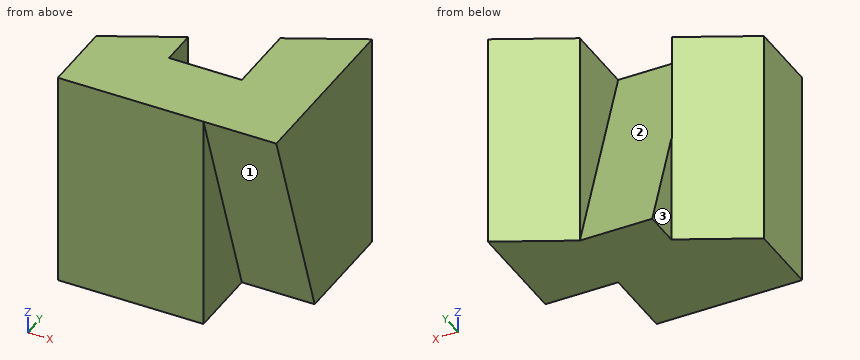
from build123d import *

# Parameters (mm, degrees)
SKETCH1_W           = 6
SKETCH1_H           = 6
BOSS_EXTRUDE1_DEPTH = 5
CUT_EXTRUDE12_DEPTH = 12
CUT_EXTRUDE13_DEPTH = 1
CUT_EXTRUDE14_DEPTH = 2


with BuildPart() as part:
    # Sketch1 → Boss-Extrude1 (new body)
    with BuildSketch(Plane(origin=(0, 0, 0), x_dir=(1, 0, 0), z_dir=(0, 1, 0))):
        Rectangle(SKETCH1_W, SKETCH1_H)
    extrude(amount=BOSS_EXTRUDE1_DEPTH)

    # Sketch11 → Cut-Extrude12 (cut)
    with BuildSketch(Plane.XY.offset(3)):
        Polygon((-3, 5), (-3, 2), (-0.98808733, 3.005956335), (-0.98808733, 4), (0.98808733, 4), (0.98808733, 3.994043665), (3, 5), align=None)
    extrude(amount=-CUT_EXTRUDE12_DEPTH, mode=Mode.SUBTRACT)

    # Sketch12 → Cut-Extrude13 (cut, symmetric)
    with BuildSketch(Plane(origin=(0, 0, 0), x_dir=(0, 0, -1), z_dir=(1, 0, 0))):
        Polygon((3, 4), (-3, 2), (-3, 3.005956335), (-3, 4), align=None)
    extrude(amount=CUT_EXTRUDE13_DEPTH, both=True, mode=Mode.SUBTRACT)

    # Sketch13 → Cut-Extrude14 (cut)
    with BuildSketch(Plane(origin=(3, 0, 0), x_dir=(0, 0, -1), z_dir=(1, 0, 0))):
        Polygon((3, 2), (-3, 0), (3, 0), align=None)
    extrude(amount=-CUT_EXTRUDE14_DEPTH, mode=Mode.SUBTRACT)


solid = part.part
Source: CAD feature listing. Evaluate the final solid. Frame: model axes, mm. Face numbers are marked on the shaded views. A direction names the side the tool comes from. Round coordinates to 2 decimals unless told otherwise and drop trailing zeros. Write each loop counter-clockwise with the first axis right and the second up, starting at its lowest first coordinate (ties: lowest second). Pieces come first, ordered by that corner, then holes. Notation, with made-up numbers: (24, 82) - (57, 82) arc R11 ccw to (57, 96) - close; hole circle Ø9 at (69, 53). An arc over 180 degrees is marked (long way). Use CSV: the item, a comma, the result in double quotes. Start each with the question number.
(1) Cut plane C-C, the plane x = 1.5. Return loops of the section in (y, z).
(2) First-contact query: pin 1 Ø1.1 at (y, z) = (3.5, -2) entering from -X; pin 2 Ø1.5 at (x, z) = (1.5, -1.5) entering from +Y (3 decimals); pin 3 Ø2 at (x, z) = (1.5, -1.5) entering from +Y. Flat tips, straight axial feed; report the tip coordinate or a pass-through.
(3) Set-up query: the marked faces 1, 2 and 3. Return all of +Z, -Z, +X, -X, +Y, -Y with unobstructed straight access to the full face (end or side cutting, diameter ignored); none if empty.
(4) Cut plane A-A, the plane y = 2.8. Return loops of the section in (x, z).
(5) Cut plane B-B, the plane z = 1.25. Return loops of the section in (x, y), and give its area (3 significant figures).
(6) Material intervals for probe 1 along X at (y, z) = (1.2, -2); probe 2 along X at (y, z) = (3.4, -2.25); probe 3 along X at (y, z) = (2.8, 2.5), sorted ascending. Write a range as [from, to].
(7) Cut plane D-D, the plane y = 0.55. Return loops of the section in (x, z), and give its area (3 significant figures).
Geometry says:
1,outline,"(0, 3) - (2, -3) - (4.25, -3) - (4.25, 3) - close"
2,pin 1,"x = -1.1"
2,pin 2,"y = 4.625"
2,pin 3,"y = 4.75"
3,face 1,"-Z, +X, -Y"
3,face 2,"+Z, +Y"
3,face 3,"+Z, -Z, -X, +Y"
4,outline,"(-1.4, -3) - (3, -3) - (3, 3) - (1, 3) - (1, 0.6) - (-1, 0.6) - (-1, 3) - (-1.4, 3) - close"
5,outline,"(-3, 0) - (1, 0) - (1, 0.58) - (3, 0.58) - (3, 5) - (1, 4) - (1, 2.58) - (-1, 2.58) - (-1, 3) - (-3, 2) - close"
5,area,"18.0 mm²"
6,probe 1,"[-3, 1]"
6,probe 2,"[-0.99, 3]"
6,probe 3,"[-1.4, -1], [1, 3]"
7,outline,"(-3, -3) - (1, -3) - (1, 1.35) - (3, 1.35) - (3, 3) - (-3, 3) - close"
7,area,"27.3 mm²"
